Verification items for this drawing (mm, ordinates from the low corner). Round coordinates to 2 decimals unless told otherwise and drop trailing zeros. Write each loop counter-clockwise with the first axis right and the second up, starting at its lowest first coordinate (ties: lowest second). Pieces come first, ordered by that corner, then holes.
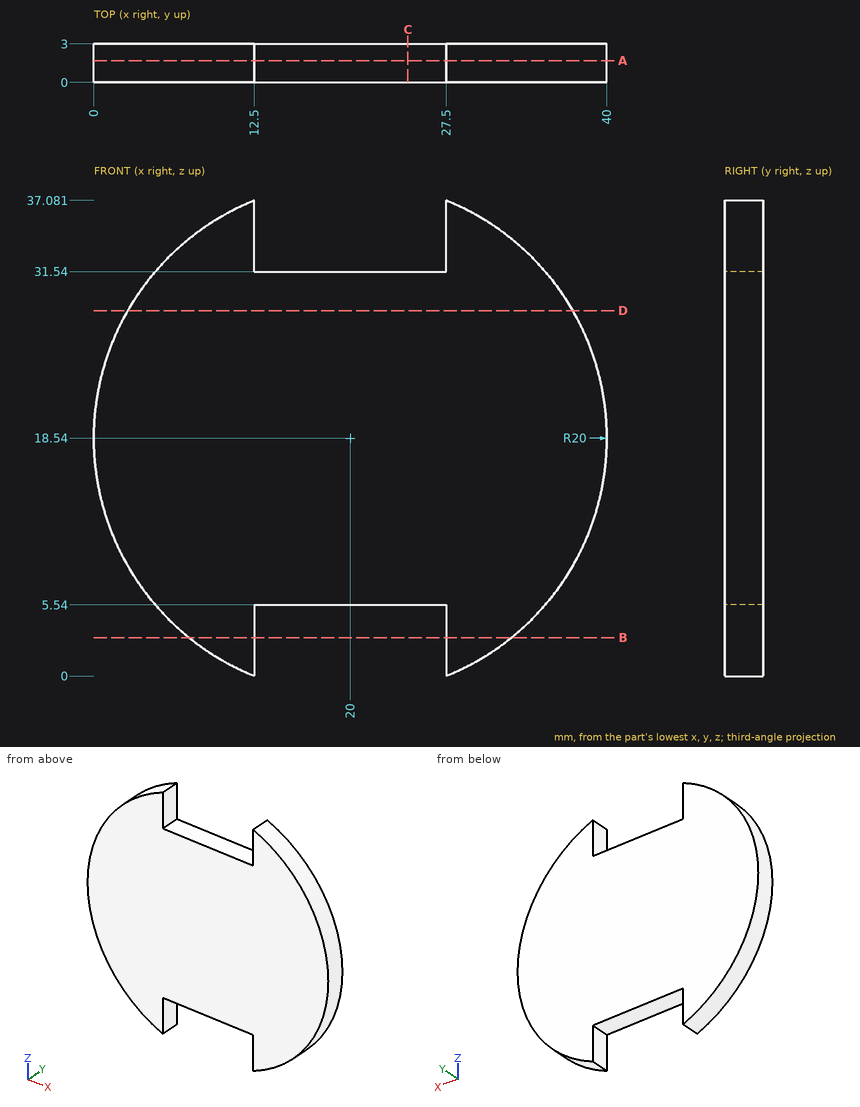
1. Depth check by flat-ended pin: pin 1 Ø1 at (x, z) = (15, 33) entering from +Y; pin 2 Ø1.5 at (y, z) = (1.5, 2) entering from +X (1 decimal); pin 3 Ø1.5 at (y, z) = (1.5, 4) entering from -X (1 decimal); pin 4 Ø0.9 at (y, z) = (2, 33) entering from -X (1 decimal). Enter the tip coordinate at first touch or a pass-through.
2. Section check A-A (y = 1.7). Record the cut outline in (x, z).
3. Scan lines: line 1 along Z through (x, y) = (19, 1.5); line 2 along Z through (x, y) = (35.5, 0.75); line 3 along X through (y, z) = (0.3, 14). Record each from-to range of solid material in increasing order.
4. Section check D-D (z = 28.5). Record the cut outline in (x, y).
5. Section check B-B (z = 3). Record the cut outline in (x, y).
6. Section check C-C (x = 24.5). Record the cut outline in (y, z).
Results below:
1. pin 1: passes through
1. pin 2: stops at x = 32.3
1. pin 3: stops at x = 5.5
1. pin 4: stops at x = 5.7
2. outline: (12.5, 0) - (12.5, 5.54) - (27.5, 5.54) - (27.5, 0) arc R20 ccw to (27.5, 37.08) - (27.5, 31.54) - (12.5, 31.54) - (12.5, 37.08) arc R20 ccw to start
3. line 1: z = 5.54 to 31.54
3. line 2: z = 5.9 to 31.18
3. line 3: x = 0.52 to 39.48
4. outline: (2.66, 0) - (37.34, 0) - (37.34, 3) - (2.66, 3) - close
5. outline: (7.41, 0) - (12.5, 0) - (12.5, 3) - (7.41, 3) - close; (27.5, 0) - (32.59, 0) - (32.59, 3) - (27.5, 3) - close
6. outline: (0, 5.54) - (3, 5.54) - (3, 31.54) - (0, 31.54) - close
